from build123d import *

# Parameters (mm, degrees)
SKETCH2_R           = 57.15
BOSS_EXTRUDE1_DEPTH = 8.35
CUT_EXTRUDE1_REACH  = 10.35
SKETCH6_R           = 3.175
SKETCH7_R           = 11.43
SKETCH7_R_2         = 1.778
CUT_EXTRUDE2_DEPTH  = 9.35
SKETCH8_R           = 4.2164
CUT_EXTRUDE3_DEPTH  = 9.35
CHAMFER1_SIZE       = 1
CIRPATTERN1_COUNT   = 6


with BuildPart() as part:
    # Sketch2 → Boss-Extrude1 (new body)
    with BuildSketch(Plane(origin=(0, 0, 0), x_dir=(1, 0, 0), z_dir=(0, 1, 0))):
        Circle(SKETCH2_R)
    extrude(amount=BOSS_EXTRUDE1_DEPTH)

    # Sketch6 → Cut-Extrude1 (cut, up to next)
    with BuildSketch(Plane(origin=(0, 8.35, 0), x_dir=(1, 0, 0), z_dir=(0, 1, 0)), mode=Mode.PRIVATE) as cut_extrude1_sk1:
        with Locations((-26.1629, -26.1629)):
            Circle(SKETCH6_R)
    cut_extrude1_tool1 = extrude(cut_extrude1_sk1.sketch, amount=-CUT_EXTRUDE1_REACH, mode=Mode.PRIVATE) & part.part
    add(cut_extrude1_tool1.solids().sort_by_distance((-26.1629, 8.35, 26.1629))[0], mode=Mode.SUBTRACT)
    # Sketch6 → Cut-Extrude1 (cut, up to next)
    with BuildSketch(Plane(origin=(0, 8.35, 0), x_dir=(1, 0, 0), z_dir=(0, 1, 0)), mode=Mode.PRIVATE) as cut_extrude1_sk2:
        with Locations((26.1629, -26.1629)):
            Circle(SKETCH6_R)
    cut_extrude1_tool2 = extrude(cut_extrude1_sk2.sketch, amount=-CUT_EXTRUDE1_REACH, mode=Mode.PRIVATE) & part.part
    add(cut_extrude1_tool2.solids().sort_by_distance((26.1629, 8.35, 26.1629))[0], mode=Mode.SUBTRACT)
    # Sketch6 → Cut-Extrude1 (cut, up to next)
    with BuildSketch(Plane(origin=(0, 8.35, 0), x_dir=(1, 0, 0), z_dir=(0, 1, 0)), mode=Mode.PRIVATE) as cut_extrude1_sk3:
        with Locations((-26.1629, 26.163103615)):
            Circle(SKETCH6_R)
    cut_extrude1_tool3 = extrude(cut_extrude1_sk3.sketch, amount=-CUT_EXTRUDE1_REACH, mode=Mode.PRIVATE) & part.part
    add(cut_extrude1_tool3.solids().sort_by_distance((-26.1629, 8.35, -26.163104))[0], mode=Mode.SUBTRACT)
    # Sketch6 → Cut-Extrude1 (cut, up to next)
    with BuildSketch(Plane(origin=(0, 8.35, 0), x_dir=(1, 0, 0), z_dir=(0, 1, 0)), mode=Mode.PRIVATE) as cut_extrude1_sk4:
        with Locations((26.1629, 26.163103615)):
            Circle(SKETCH6_R)
    cut_extrude1_tool4 = extrude(cut_extrude1_sk4.sketch, amount=-CUT_EXTRUDE1_REACH, mode=Mode.PRIVATE) & part.part
    add(cut_extrude1_tool4.solids().sort_by_distance((26.1629, 8.35, -26.163104))[0], mode=Mode.SUBTRACT)

    # Sketch7 → Cut-Extrude2 (cut, through all)
    with BuildSketch(Plane(origin=(0, 8.35, 0), x_dir=(1, 0, 0), z_dir=(0, 1, 0))):
        with Locations((32, 0)):
            Circle(SKETCH7_R)
        with Locations((18.54, -13.464)):
            Circle(SKETCH7_R_2)
        with Locations((18.54, 13.46)):
            Circle(SKETCH7_R_2)
        with Locations((45.46, 13.46)):
            Circle(SKETCH7_R_2)
        with Locations((45.46, -13.464)):
            Circle(SKETCH7_R_2)
    extrude(amount=-CUT_EXTRUDE2_DEPTH, mode=Mode.SUBTRACT)

    # Sketch8 → Cut-Extrude3 (cut, through all)
    with BuildSketch(Plane(origin=(0, 8.35, 0), x_dir=(1, 0, 0), z_dir=(0, 1, 0))):
        Circle(SKETCH8_R)
        with BuildLine():
            Line((-39.95, 5.249761899), (-39.95, -5.249761899))
            ThreePointArc((-39.95, -5.249761899), (-18.75, 0), (-39.95, 5.249761899))
        make_face()
    extrude(amount=-CUT_EXTRUDE3_DEPTH, mode=Mode.SUBTRACT)

    # Chamfer1
    chamfer1_edges = [part.edges().sort_by_distance(p)[0] for p in [
        (-57.15, 0, 0),
        (-57.15, 8.35, 0),
    ]]
    chamfer(chamfer1_edges, length=CHAMFER1_SIZE)

    # Sketch11 → #6-32 Tapped Hole1 (revolve, cut)
    with BuildSketch(Plane(origin=(0, 4.175, 57.15), x_dir=(0, -1, 0), z_dir=(1, 0, 0))):
        Polygon((0, 0), (0, 13.81269403), (1.35255, 13), (1.35255, 0), align=None)
    f_6_32_tapped_hole1 = revolve(axis=Axis((0, 4.175, 63.5), (0, 0, -1)), mode=Mode.SUBTRACT)

    # CirPattern1: #6-32 Tapped Hole1 ×6 about axis
    cirpattern1_axis = Axis((0, 1, 0), (0, 1, 0))
    for i in range(1, CIRPATTERN1_COUNT):
        add(f_6_32_tapped_hole1.rotate(cirpattern1_axis, i * 360 / CIRPATTERN1_COUNT), mode=Mode.SUBTRACT)


solid = part.part
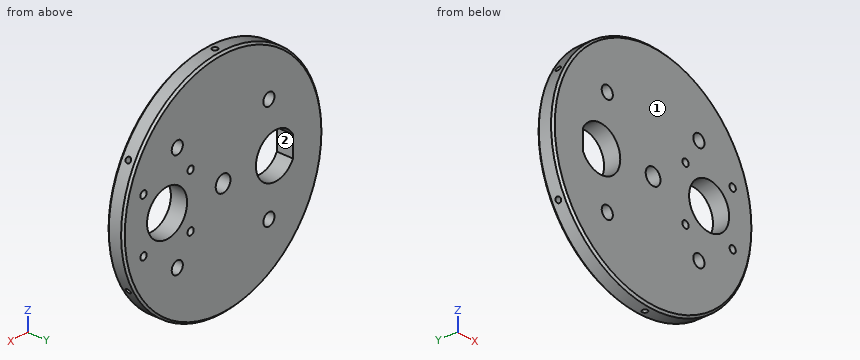
Read the model definition and answer for the solid it produces. Units are mm, in the model's axes. Face numbers are marked on the shaded views. Round coordinates to 2 decimals unless told otherwise and drop trailing zeros. Order: outer loops, then holes, each group sorted by start corner. A loop starts at its lowest first (then second) coordinate and runs counter-clockwise, first axis right, second up.
1) The part is cut by section A-A on z = 0. Write down the section's boundary in (x, y), plus the area to 3 significant figures.
2) Flat-ended cylindrical pins translate along their axes: pin 1 (2 mm diameter, centred on y = 4.5, z = 4.5, fed in from -X); pin 2 (18.5 mm diameter, centred on x = 32, z = 0, fed in from -Y); pin 3 (5 mm diameter, centred on y = 2.5, z = 27.5, fed in from -X); pin 4 (5 mm diameter, centred on y = 7.5, z = -39, fed in from +X). Find the tip coordinate at first contact, or state that the pin passes through.
3) The mould has two halves that part along X. Classify the marked faces 1 and 2: released by +X, released by -X, zero draft, split by the parting line, or undercut.
4) Straight lines are drawn through the part: L1, parallel to X at y = 3.75, z = 12.5; L2, parallel to Z at x = 24, y = 5; L3, parallel to X at y = 1.5, z = 28.5. For each, find the intervals that lie inside material, in ascending order.
5) The part is cut by section B-B on x = 45.46. Give the number of separate pieces and of enclosed holes in the cut face, plus the area to 3 significant figures.
Resolved:
1. outline: (-57.15, 1) - (-56.15, 0) - (-39.95, 0) - (-39.95, 8.35) - (-56.15, 8.35) - (-57.15, 7.35) - close; (-18.75, 0) - (-4.22, 0) - (-4.22, 8.35) - (-18.75, 8.35) - close; (4.22, 0) - (20.57, 0) - (20.57, 8.35) - (4.22, 8.35) - close; (43.43, 0) - (56.15, 0) - (57.15, 1) - (57.15, 7.35) - (56.15, 8.35) - (43.43, 8.35) - close
1. area: 514 mm2
2. pin 1: stops at x = -57.04
2. pin 2: passes through
2. pin 3: stops at x = -51.39
2. pin 4: stops at x = 43.97
3. face 1: zero draft
3. face 2: undercut
4. L1: x = -55.77 to 17.05, 20.03 to 43.97, 46.95 to 55.77
4. L2: z = -51.87 to -28.49, -23.84 to -8.16, 8.16 to 23.84, 28.49 to 51.87
4. L3: x = -49.54 to -28.31, -24.01 to 24.01, 28.31 to 49.54
5. separate pieces: 3
5. enclosed holes: 2
5. area: 502 mm2
